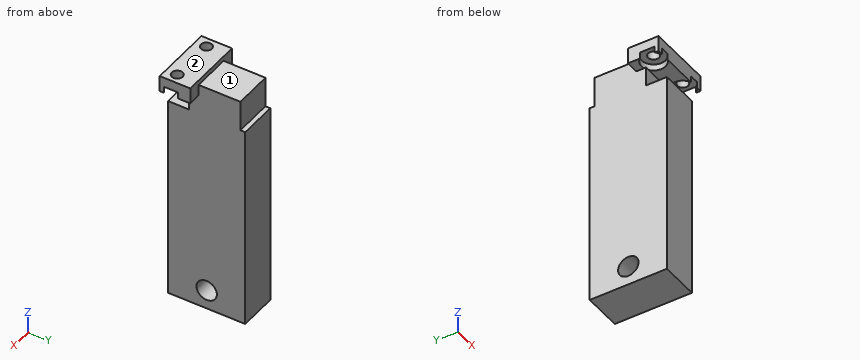
```python
from build123d import *

# Parameters (mm, degrees)
FIVE_MM_ATTACHMENT_FOOT_START                      = -5
SKETCH1_W                                          = 20
SKETCH1_H                                          = 9.5
SKETCH1_R                                          = 1.7
FIVE_MM_ATTACHMENT_FOOT_DEPTH                      = 5
DEEP_ACTUATOR_WEB_START                            = -69
SKETCH2_W                                          = 12
SKETCH2_H                                          = 24
DEEP_ACTUATOR_WEB_DEPTH                            = 67.5
QUARTER20_AXIAL_THREAD_MAJOR_ENVELOPE_DEPTH        = 90.516758208
QUARTER20_AXIAL_THREAD_MAJOR_ENVELOPE_DEPTH_BACK   = 90.516758208
SKETCH3_R                                          = 3.175
BENCH_X_BORE_LOWER_LIGAMENT_START                  = -75
SKETCH4_W                                          = 12
SKETCH4_H                                          = 24
BENCH_X_BORE_LOWER_LIGAMENT_DEPTH                  = 6.01
BENCH_COMPLETE_QUARTER20_MAJOR_ENVELOPE_DEPTH      = 95.21915941
BENCH_COMPLETE_QUARTER20_MAJOR_ENVELOPE_DEPTH_BACK = 95.21915941
SKETCH5_R                                          = 3.175
FIXED_BASE_WINDOW_RELIEF_DEPTH                     = 95.21915941
FIXED_BASE_WINDOW_RELIEF_DEPTH_BACK                = 95.21915941
SKETCH6_W                                          = 6
SKETCH6_H                                          = 7
SKETCH6_W_2                                        = 10
SKETCH6_H_2                                        = 2
XDROP_M3_THROUGH_RECUT_START                       = -5.5
SKETCH7_R                                          = 1.7
XDROP_M3_THROUGH_RECUT_DEPTH                       = 5.5
SKETCH8_R                                          = 3.75
XDROP_M3_BOTTOM_COUNTERBORE_H2_DEPTH               = 2


with BuildPart() as part:
    # Sketch1 → Five_mm_Attachment_Foot (new body)
    with BuildSketch(Plane.XY.offset(FIVE_MM_ATTACHMENT_FOOT_START)):
        with Locations((-20, 29.25)):
            Rectangle(SKETCH1_W, SKETCH1_H)
        with Locations((-27, 28)):
            Circle(SKETCH1_R, mode=Mode.SUBTRACT)
        with Locations((-13, 28)):
            Circle(SKETCH1_R, mode=Mode.SUBTRACT)
    extrude(amount=FIVE_MM_ATTACHMENT_FOOT_DEPTH)

    # Sketch2 → Deep_Actuator_Web (add)
    with BuildSketch(Plane.XY.offset(DEEP_ACTUATOR_WEB_START)):
        with Locations((-20, 36.5)):
            Rectangle(SKETCH2_W, SKETCH2_H)
    extrude(amount=DEEP_ACTUATOR_WEB_DEPTH)

    # Sketch3 → Quarter20_Axial_Thread_Major_Envelope (cut, two sides: drawn at the far end of the back side and taken through both)
    with BuildSketch(Plane(origin=(0, 0, 0), x_dir=(0, 0, -1), z_dir=(1, 0, 0)).offset(-QUARTER20_AXIAL_THREAD_MAJOR_ENVELOPE_DEPTH_BACK)):
        with Locations((69, 36.5)):
            Circle(SKETCH3_R)
    extrude(amount=QUARTER20_AXIAL_THREAD_MAJOR_ENVELOPE_DEPTH + QUARTER20_AXIAL_THREAD_MAJOR_ENVELOPE_DEPTH_BACK, mode=Mode.SUBTRACT)

    # Sketch4 → Bench_X_Bore_Lower_Ligament (add)
    with BuildSketch(Plane.XY.offset(BENCH_X_BORE_LOWER_LIGAMENT_START)):
        with Locations((-20, 36.5)):
            Rectangle(SKETCH4_W, SKETCH4_H)
    extrude(amount=BENCH_X_BORE_LOWER_LIGAMENT_DEPTH)

    # Sketch5 → Bench_Complete_Quarter20_Major_Envelope (cut, two sides: drawn at the far end of the back side and taken through both)
    with BuildSketch(Plane(origin=(0, 0, 0), x_dir=(0, 0, -1), z_dir=(1, 0, 0)).offset(-BENCH_COMPLETE_QUARTER20_MAJOR_ENVELOPE_DEPTH_BACK)):
        with Locations((69, 36.5)):
            Circle(SKETCH5_R)
    extrude(amount=BENCH_COMPLETE_QUARTER20_MAJOR_ENVELOPE_DEPTH + BENCH_COMPLETE_QUARTER20_MAJOR_ENVELOPE_DEPTH_BACK, mode=Mode.SUBTRACT)

    # Sketch6 → Fixed_Base_Window_Relief (cut, two sides: drawn at the far end of the back side and taken through both)
    with BuildSketch(Plane(origin=(0, 0, 0), x_dir=(0, 0, -1), z_dir=(1, 0, 0)).offset(-FIXED_BASE_WINDOW_RELIEF_DEPTH_BACK)):
        with Locations((8, 27.5)):
            Rectangle(SKETCH6_W, SKETCH6_H)
        with Locations((6, 48)):
            Rectangle(SKETCH6_W_2, SKETCH6_H_2)
    extrude(amount=FIXED_BASE_WINDOW_RELIEF_DEPTH + FIXED_BASE_WINDOW_RELIEF_DEPTH_BACK, mode=Mode.SUBTRACT)

    # Sketch7 → XDrop_M3_Through_Recut (cut)
    with BuildSketch(Plane.XY.offset(XDROP_M3_THROUGH_RECUT_START)):
        with Locations((-27, 28)):
            Circle(SKETCH7_R)
        with Locations((-13, 28)):
            Circle(SKETCH7_R)
    extrude(amount=XDROP_M3_THROUGH_RECUT_DEPTH, mode=Mode.SUBTRACT)

    # Sketch8 → XDrop_M3_Bottom_Counterbore_H2 (cut)
    with BuildSketch(Plane(origin=(0, 0, -5), x_dir=(-1, 0, 0), z_dir=(0, 0, -1))):
        with Locations((27, 28)):
            Circle(SKETCH8_R)
        with Locations((13, 28)):
            Circle(SKETCH8_R)
    extrude(amount=-XDROP_M3_BOTTOM_COUNTERBORE_H2_DEPTH, mode=Mode.SUBTRACT)


solid = part.part
```
The model under review builds one solid part; all positions refer to its coordinate system, in mm. Face numbers are marked on the shaded views. A direction names the side the tool comes from. Round coordinates to 2 decimals unless told otherwise and drop trailing zeros. Loops run counter-clockwise (first coordinate to the right, second up) from the corner with the lowest first, then second, coordinate; pieces in that order, holes last.
Item 1: Take a section at C-C (x = -27). Write out the cut boundary in (y, z).
Determined:
outline: (24.5, -3) - (26.3, -3) - (26.3, 0) - (24.5, 0) - close; (29.7, -3) - (31.75, -3) - (31.75, -5) - (34, -5) - (34, 0) - (29.7, 0) - close
Item 2: Take a section at B-B (y = 28). Write out the cut boundary in (x, z), then the cut area to 3 significant figures.
Determined:
outline: (-30, -3) - (-28.7, -3) - (-28.7, 0) - (-30, 0) - close; (-26, -75) - (-14, -75) - (-14, -11) - (-26, -11) - close; (-25.3, -3) - (-23.25, -3) - (-23.25, -5) - (-16.75, -5) - (-16.75, -3) - (-14.7, -3) - (-14.7, 0) - (-25.3, 0) - close; (-11.3, -3) - (-10, -3) - (-10, 0) - (-11.3, 0) - close
area: 821 mm2
Item 3: Take a section at D-D (y = 36.5). Write out the cut boundary in (x, z) (3 decimals).
Determined:
outline: (-26, -75) - (-14, -75) - (-14, -72.175) - (-26, -72.175) - close; (-26, -65.825) - (-14, -65.825) - (-14, -1.5) - (-26, -1.5) - close
Item 4: Clearance check with flat-ended pins moving along their axes: pin 1 Ø7 at (y, z) = (40, -20) entering from +X; pin 2 Ø2.5 at (x, y) = (-27, 28) entering from +Z; pin 3 Ø2 at (y, z) = (31, -19) entering from -X. State where each tip first meets the part, or that it passes through.
Determined:
pin 1: stops at x = -14
pin 2: stops at z = -11
pin 3: stops at x = -26
Item 5: For the marked faces 1 and 2, list the 3-axis set-ups (+Z, -Z, +X, -X, +Y, -Y) from which the entire face can be reached by the end or side of a thin tool; tool diameter is ignored.
Determined:
face 1: +Z, +X, -X, +Y
face 2: +Z, +X, -X, +Y, -Y
Item 6: Take a section at A-A (z = -69). Write out the cut boundary in (x, y) (3 decimals), then the cut area to 3 significant figures.
Determined:
outline: (-26, 24.5) - (-14, 24.5) - (-14, 33.325) - (-26, 33.325) - close; (-26, 39.675) - (-14, 39.675) - (-14, 48.5) - (-26, 48.5) - close
area: 212 mm2
Item 7: For line 1 (X direction, y = 28, z = -1.6); line 2 (Y direction, x = -18.25, z = -69) (3 decimals); line 3 (Y direction, x = -13, z = -0.9), list the stretches that pass through material, from the lowest coordinate up.
Determined:
line 1: x = -30 to -28.7, -25.3 to -14.7, -11.3 to -10
line 2: y = 24.5 to 33.325, 39.675 to 48.5
line 3: y = 24.5 to 26.3, 29.7 to 34
